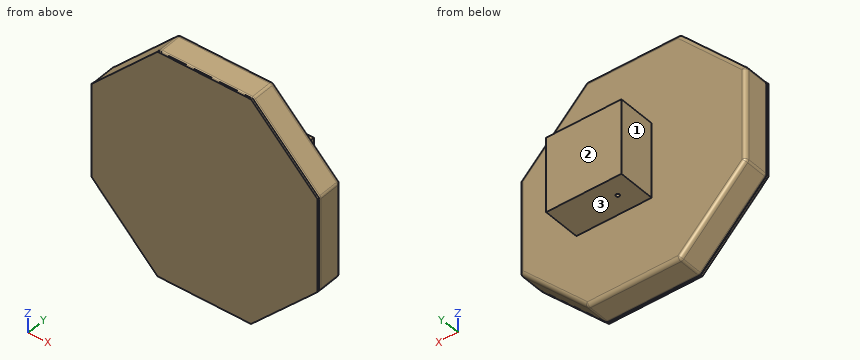
```python
from build123d import *

# Parameters (mm, degrees)
BOSS_EXTRUDE2_DEPTH = 15
SKETCH3_W           = 40
SKETCH3_H           = 40
BOSS_EXTRUDE3_DEPTH = 20
FILLET2_R           = 2
SKETCH4_R           = 1
CUT_EXTRUDE1_DEPTH  = 40
BOSS_EXTRUDE4_DEPTH = 1


with BuildPart() as part:
    # Sketch2 → Boss-Extrude2 (new body)
    with BuildSketch(Plane(origin=(0, 0, 0), x_dir=(1, 0, 0), z_dir=(0, 1, 0))):
        Polygon((-60, -24.852813742), (-24.852813742, -60.262270904), (24.852813742, -60.262270904), (60.262270904, -24.852813742), (60.262270904, 24.852813742), (24.852813742, 60.262270904), (-24.852813742, 60.262270904), (-60, 24.852813742), align=None)
    extrude(amount=BOSS_EXTRUDE2_DEPTH)

    # Sketch3 → Boss-Extrude3 (add)
    with BuildSketch(Plane(origin=(0, 15, 0), x_dir=(1, 0, 0), z_dir=(0, 1, 0))):
        with Locations((10, 0)):
            Rectangle(SKETCH3_W, SKETCH3_H)
    extrude(amount=BOSS_EXTRUDE3_DEPTH)

    # Fillet2
    fillet2_edges = [part.edges().sort_by_distance(p)[0] for p in [
        (0, 0, 60.262270904),
        (-42.426406871, 0, 42.557542323),
        (-60, 0, 0),
        (-42.426406871, 0, -42.557542323),
        (-42.426406871, 15, 42.557542323),
        (-24.852813742, 7.5, -60.262270904),
        (24.852813742, 7.5, -60.262270904),
        (60.262270904, 7.5, -24.852813742),
        (60.262270904, 7.5, 24.852813742),
        (24.852813742, 7.5, 60.262270904),
        (-24.852813742, 7.5, 60.262270904),
        (-60, 7.5, 24.852813742),
        (-60, 7.5, -24.852813742),
        (0, 15, 60.262270904),
        (42.557542323, 15, 42.557542323),
        (60.262270904, 15, 0),
        (42.557542323, 15, -42.557542323),
        (0, 15, -60.262270904),
        (-42.426406871, 15, -42.557542323),
        (0, 0, -60.262270904),
        (-60, 15, 0),
        (42.557542323, 0, -42.557542323),
        (60.262270904, 0, 0),
        (42.557542323, 0, 42.557542323),
    ]]
    fillet(fillet2_edges, radius=FILLET2_R)

    # Sketch4 → Cut-Extrude1 (cut)
    with BuildSketch(Plane.XY.offset(20)):
        with Locations((0, 25)):
            Circle(SKETCH4_R)
    extrude(amount=-CUT_EXTRUDE1_DEPTH, mode=Mode.SUBTRACT)

    # Sketch1 → Boss-Extrude4 (add)
    with BuildSketch(Plane(origin=(0, 0, 0), x_dir=(1, 0, 0), z_dir=(0, 1, 0))):
        Polygon((-60.131135452, -24.852813742), (-24.983949194, -60.262270904), (24.72167829, -60.262270904), (60.131135452, -24.852813742), (60.131135452, 24.852813742), (24.72167829, 60.262270904), (-24.983949194, 60.262270904), (-60.131135452, 24.852813742), align=None)
    extrude(amount=BOSS_EXTRUDE4_DEPTH)


solid = part.part
```
Input: part model. Units: mm. Frame: model coordinates. Face numbers are marked on the shaded views. A direction names the side the tool comes from. Round coordinates to 2 decimals unless told otherwise and drop trailing zeros. Loops run counter-clockwise (first coordinate to the right, second up) from the corner with the lowest first, then second, coordinate; pieces in that order, holes last. Notation, with made-up numbers: (55.25, 8.5) -> (78.25, 8.5) arc R18 cw to (78.25, 36.5) -> close; hole circle Ø9 at (15, 61). An arc over 180 degrees is marked (long way). Write each question's results on one line, items separated by ' | '.
1. Section D-D (x = 21.5). Return loops of the section in (y, z), and give its area (3 significant figures).
Geometry results:
outline: (0, -60.26) -> (1, -60.26) -> (1, -59.99) arc R2 ccw to (2, -60.26) -> (13, -60.26) arc R2 ccw to (15, -58.26) -> (15, -20) -> (35, -20) -> (35, 20) -> (15, 20) -> (15, 58.26) arc R2 ccw to (13, 60.26) -> (2, 60.26) arc R2 ccw to (1, 59.99) -> (1, 60.26) -> (0, 60.26) -> close | area: 2,610 mm2
2. First-contact query: P1, Ø8, axis at x = 11.5, y = 18, coming from the -Z side; P2, Ø16, axis at y = 28.5, z = 7.5, coming from the -X side; P3, Ø8, axis at y = 13.5, z = -11.5, coming from the -X side; P4, Ø8, axis at y = 21, z = -45, coming from the -X side. Flat tips, straight axial feed; report the tip coordinate or a pass-through.
Geometry results:
P1: z = -59.99 | P2: x = -10 | P3: x = -60 | P4: through
3. Section A-A (z = -8). Return loops of the section in (x, y).
Geometry results:
outline: (-60.13, 0) -> (60.13, 0) -> (60.13, 1) -> (59.99, 1) arc R2 ccw to (60.26, 2) -> (60.26, 13) arc R2 ccw to (58.26, 15) -> (30, 15) -> (30, 35) -> (-10, 35) -> (-10, 15) -> (-58, 15) arc R2 ccw to (-60, 13) -> (-60, 2) arc R2 ccw to (-59.73, 1) -> (-60.13, 1) -> close; hole circle Ø2 at (0, 25)
4. Section B-B (x = -19). Return loops of the section in (y, z), and give its area (3 significant figures).
Geometry results:
outline: (0, -60.26) -> (1, -60.26) -> (1, -59.99) arc R2 ccw to (2, -60.26) -> (13, -60.26) arc R2 ccw to (15, -58.26) -> (15, 58.26) arc R2 ccw to (13, 60.26) -> (2, 60.26) arc R2 ccw to (1, 59.99) -> (1, 60.26) -> (0, 60.26) -> close | area: 1,810 mm2
5. Ray query, line 1 (Y direction, x = 0, z = 10.5); line 2 (Y direction, x = -32, z = -1); line 3 (X direction, y = 19, z = 13). Return the intervals inside material, ascending. Write a range as from..to.
Geometry results:
line 1: 0..24, 26..35 | line 2: 0..15 | line 3: -10..30
6. Set-up query: the marked faces 1, 2 and 3. Return all of +Z, -Z, +X, -X, +Y, -Y with unobstructed straight access to the full face (end or side cutting, diameter ignored); none if empty.
Geometry results:
face 1: +Z, -Z, -X, +Y | face 2: +Z, -Z, +X, -X, +Y | face 3: -Z, +X, -X, +Y
7. Section C-C (y = 4). Return loops of the section in (x, z), and give its area (3 significant figures).
Geometry results:
outline: (-60, -24.03) arc R2 ccw to (-59.42, -25.44) -> (-25.44, -59.67) arc R2 ccw to (-24.02, -60.26) -> (24.02, -60.26) arc R2 ccw to (25.44, -59.68) -> (59.68, -25.44) arc R2 ccw to (60.26, -24.02) -> (60.26, 24.02) arc R2 ccw to (59.68, 25.44) -> (25.44, 59.68) arc R2 ccw to (24.02, 60.26) -> (-24.02, 60.26) arc R2 ccw to (-25.44, 59.67) -> (-59.42, 25.44) arc R2 ccw to (-60, 24.03) -> close | area: 12,000 mm2
